from build123d import *

# Parameters (mm, degrees)
SKETCH1_W           = 43
SKETCH1_H           = 20
BOSS_EXTRUDE1_DEPTH = 1
SKETCH2_R           = 5
BOSS_EXTRUDE2_DEPTH = 7
FILLET1_R           = 2
FILLET2_R           = 1


with BuildPart() as part:
    # Sketch1 → Boss-Extrude1 (new body, symmetric)
    with BuildSketch(Plane.XY):
        Rectangle(SKETCH1_W, SKETCH1_H)
    extrude(amount=BOSS_EXTRUDE1_DEPTH, both=True)

    # Sketch2 → Boss-Extrude2 (add)
    with BuildSketch(Plane.XY.offset(-1)):
        with Locations((-12.5, 0)):
            Circle(SKETCH2_R)
        with Locations((12.5, 0)):
            Circle(SKETCH2_R)
    extrude(amount=-BOSS_EXTRUDE2_DEPTH)

    # Fillet1
    fillet1_edges = [part.edges().sort_by_distance(p)[0] for p in [
        (-17.5, 0, -1),
        (7.5, 0, -1),
    ]]
    fillet(fillet1_edges, radius=FILLET1_R)

    # Fillet2
    fillet2_edges = [part.edges().sort_by_distance(p)[0] for p in [
        (21.5, -10, 0),
        (-21.5, -10, 0),
        (-21.5, 10, 0),
        (21.5, 10, 0),
    ]]
    fillet(fillet2_edges, radius=FILLET2_R)


solid = part.part
Here's how the part is built. I have some questions about the finished solid (model axes, mm). A direction names the side the tool comes from. Coordinates: 2 decimals unless noted, no trailing zeros. Loops run counter-clockwise (first coordinate to the right, second up) from the corner with the lowest first, then second, coordinate; pieces in that order, holes last.
1. Imagine slicing it at A-A, the plane x = -12.5. Please give me the cut outline in (y, z), and give its area (3 significant figures).
2. Imagine slicing it at C-C, the plane z = -3.75. Please give me the cut outline in (x, y).
3. Imagine slicing it at D-D, the plane x = -4. Please give me the cut outline in (y, z).
4. Imagine slicing it at B-B, the plane y = 0. Please give me the cut outline in (x, z).
5. I need wall thicknesses on L1, parallel to Z at x = -15, y = 6.75; L2, parallel to X at y = -1.25, z = -1.25; L3, parallel to X at y = -2, z = -3.25. Which ranges of each line are inside material? Lowest first, please.
6. If we mould it in two halves opening along X, with no side actions, what happens to faces 3 (the cylindrical face through (21.199, -9.715, 0.014)), 4 (the cylindrical face through (17.27, 1.5, -5.46)), 5 (the flat face through (-13, 0, -8)), 6 (the flat face through (0, 0, -1))? For each: pulls with the +X half, pulls with the -X half, needs draft (parallel to the pull), parting line crosses it, or undercut.
7. For P1, Ø1, axis at x = 10, z = -6, coming from the -Y side; P2, Ø12, axis at x = 0, y = -4, coming from the -Z side; P3, Ø3, axis at y = 6, z = -2, coming from the -X side; P4, Ø1, axis at x = -14, z = -4.5, coming from the +Y side, each with a flat end and sliding along its axis, tell me the tip position at first contact or that it passes through.
8. For faces 1 (the cylindrical face through (-7.73, 1.5, -5.46)), 2 (the flat face through (21.5, 0, 0)), which set-ups out of +Z, -Z, +X, -X, +Y, -Y let a thin tool reach every point of the face, with its end or its side?
Taken from the geometry:
1. outline: (-10, -1) - (-7, -1) arc R2 cw to (-5, -3) - (-5, -8) - (5, -8) - (5, -3) arc R2 cw to (7, -1) - (10, -1) - (10, 1) - (-10, 1) - close
1. area: 112 mm2
2. outline: circle Ø10 at (-12.5, 0); circle Ø10 at (12.5, 0)
3. outline: (-10, -1) - (10, -1) - (10, 1) - (-10, 1) - close
4. outline: (-21.5, -1) - (-19.5, -1) arc R2 cw to (-17.5, -3) - (-17.5, -8) - (-7.5, -8) - (-7.5, -3) arc R2 cw to (-5.5, -1) - (5.5, -1) arc R2 cw to (7.5, -3) - (7.5, -8) - (17.5, -8) - (17.5, -3) arc R2 cw to (19.5, -1) - (21.5, -1) - (21.5, 1) - (-21.5, 1) - close
5. L1: z = -1 to 1
5. L2: x = -18.4 to -6.6, 6.6 to 18.4
5. L3: x = -17.08 to -7.92, 7.92 to 17.08
6. face 3: pulls with the +X half
6. face 4: undercut
6. face 5: needs draft
6. face 6: undercut
7. P1: stops at y = -4.58
7. P2: stops at z = -1
7. P3: stops at x = -21.5
7. P4: stops at y = 4.9
8. face 1: -Z
8. face 2: +Z, -Z, +X, +Y, -Y
